The model under review builds one solid part; all positions refer to its coordinate system, in mm. A direction names the side the tool comes from. Coordinates: 2 decimals unless noted, no trailing zeros. Write each loop counter-clockwise with the first axis right and the second up, starting at its lowest first coordinate (ties: lowest second). Pieces come first, ordered by that corner, then holes.
```python
from build123d import *

# Parameters (mm, degrees)
F0_R     = 73.025
F1_DEPTH = 57.15
F3_DEPTH = 44.45
F4_R     = 5.08
F5_R     = 5.08


with BuildPart() as f1:
    # F0 (on Top) → F1 (new body)
    with BuildSketch(Plane.XY):
        Circle(F0_R)
    extrude(amount=F1_DEPTH)

    # F2 (on face) → F3 (cut)
    with BuildSketch(Plane.XY.offset(57.15)):
        with BuildLine():
            Line((-9.652, 0), (-9.652, 59.5478338901))
            ThreePointArc((-9.652, 59.5478338901), (-60.325, 0), (-9.652, -59.5478338901))
            Line((-9.652, -59.5478338901), (-9.652, 0))
        make_face()
        with BuildLine():
            ThreePointArc((9.652, -59.5478338901), (45.9421512611, -39.0950682631), (60.325, 0))
            ThreePointArc((60.325, 0), (45.9421512611, 39.0950682631), (9.652, 59.5478338901))
            Line((9.652, 59.5478338901), (9.652, 0))
            Line((9.652, 0), (9.652, -59.5478338901))
        make_face()
    extrude(amount=-F3_DEPTH, mode=Mode.SUBTRACT)

    # F4
    f4_edges = [f1.edges().sort_by_distance(p)[0] for p in [
        (-9.652, 59.547834, 34.925),
    ]]
    fillet(f4_edges, radius=F4_R)

    # F5
    f5_edges = [f1.edges().sort_by_distance(p)[0] for p in [
        (9.652, 59.547834, 34.925),
        (9.652, -59.547834, 34.925),
        (-9.652, -59.547834, 34.925),
    ]]
    fillet(f5_edges, radius=F5_R)


solid = f1.part
```
Item 1: For pin 1 (6 mm diameter, centred on x = -38, z = 32, fed in from +Y); pin 2 (2 mm diameter, centred on y = -55.5, z = 30.5, fed in from +X); pin 3 (5 mm diameter, centred on x = 53, z = 39, fed in from +Y), all flat-tipped, find the tip position at first contact; note any pin that passes through.
Solved:
pin 1: stops at y = 64.09
pin 2: stops at x = 48.6
pin 3: stops at y = 52.75
Item 2: To check wall thickness, follow line 1 along X through (y, z) = (-36, 30.5); line 2 along X through (y, z) = (-23.5, 19); line 3 along Z through (x, y) = (-56.5, -1.5). State the ranges of each line that lie inside material, in increasing order.
Solved:
line 1: x = -63.53 to -48.41, -9.65 to 9.65, 48.41 to 63.53
line 2: x = -69.14 to -55.56, -9.65 to 9.65, 55.56 to 69.14
line 3: z = 0 to 12.7
Item 3: Take a section at B-B, the plane y = 42.5. Write out the cut boundary in (x, z).
Solved:
outline: (-59.38, 0) - (59.38, 0) - (59.38, 57.15) - (42.81, 57.15) - (42.81, 12.7) - (9.65, 12.7) - (9.65, 57.15) - (-9.65, 57.15) - (-9.65, 12.7) - (-42.81, 12.7) - (-42.81, 57.15) - (-59.38, 57.15) - close
Item 4: Machinability: for faces 1 (the face through (-11.71, 57.33, 34.61)), 2 (the face through (-6, 0, 57.15)), which of the approach directions +Z, -Z, +X, -X, +Y, -Y give a long, thin tool a straight path to every point of the face, cutting with its end or side? Answer none if there is none.
Solved:
face 1: +Z
face 2: +Z, +X, -X, +Y, -Y
Item 5: Take a section at A-A, the plane z = 45. Write out the cut boundary in (x, y) (3 decimals).
Solved:
outline: circle Ø146.05 at (0, 0); hole (-16.087, -58.141) arc R5.08 ccw to (-9.652, -53.245) - (-9.652, 53.245) arc R5.08 ccw to (-16.087, 58.141) arc R60.325 ccw to start; hole (9.652, -53.245) arc R5.08 ccw to (16.087, -58.141) arc R60.325 ccw to (16.087, 58.141) arc R5.08 ccw to (9.652, 53.245) - close
Item 6: Take a section at C-C, the plane x = 44. Write out the cut boundary in (y, z), plus the area to 3 significant figures.
Solved:
outline: (-58.28, 0) - (58.28, 0) - (58.28, 57.15) - (41.27, 57.15) - (41.27, 12.7) - (-41.27, 12.7) - (-41.27, 57.15) - (-58.28, 57.15) - close
area: 2,990 mm2
Item 7: Mouldability with a two-part tool opening along Y and no side actions: class faces 3 (the face through (-1, 1, 0)), 4 (the face through (29, 1, 12.7)), 5 (the face through (69.653, 21.935, 28.175)) as pulls with the +Y half, pulls with the -Y half, needs draft (parallel to the pull), parting line crosses it, or undercut.
Solved:
face 3: needs draft
face 4: undercut
face 5: parting line crosses it
Item 8: Take a section at D-D, the plane z = 7.5. Write out the cut boundary in (x, y) (3 decimals), plus the area to 3 significant figures.
Solved:
outline: circle Ø146.05 at (0, 0)
area: 16,800 mm2
